CAD build for the part. Positions are in the model's coordinates, mm. Face numbers are marked on the shaded views. Give positions to 0.01 mm unless a question says otherwise; leave off trailing zeros. Order: outer loops, then holes, each group sorted by start corner. A loop starts at its lowest first (then second) coordinate and runs counter-clockwise, first axis right, second up.
Item 1: Wall check: L1, parallel to Z at x = -32.5, y = 0.8; L2, parallel to Z at x = 59.5, y = 0.85; L3, parallel to Z at x = 40, y = 1.95. Give the ranges that are in metal, low to high.
Item 2: Band-saw the part on A-A on z = -5.5. Give the cut face in (x, y), plus the area to 3 significant figures.
Item 3: Band-saw the part on D-D on x = 61. Give the cut face in (y, z).
Item 4: Band-saw the part on B-B on x = -25. Give the cut face in (y, z), plus the area to 3 significant figures.
Item 5: Flat gauge pin, fed straight in: P1, Ø0.6, axis at x = 65.5, y = 1, coming from the +Z side. Where does the tip first touch, or does it go through?
Item 6: Band-saw the part on C-C on y = 0.35. Give the cut face in (x, z).
Item 7: Two-plate mould, pull along Y, no slides. Class the marked faces 1 and 2: released by +Y, released by -Y, zero draft, split by the parting line, or undercut.
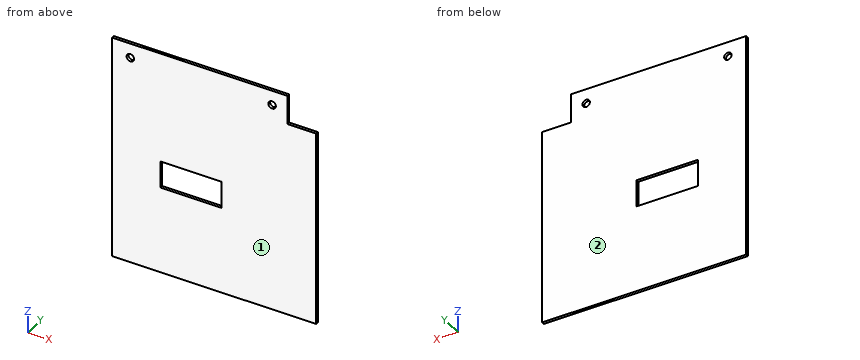
```python
from build123d import *

# Parameters (mm, degrees)
P_IDAT_VYSUNUT_M1_DEPTH  = 2
SKICA2_W                 = 42.685297449
SKICA2_H                 = 18.521827687
ODEBRAT_VYSUNUT_M1_DEPTH = 2
SKICA3_R                 = 2.6
ODEBRAT_VYSUNUT_M2_DEPTH = 2


with BuildPart() as part:
    # Skica1 → Přidat vysunutím1 (new body)
    with BuildSketch(Plane(origin=(0, 0, 0), x_dir=(1, 0, 0), z_dir=(0, 1, 0))):
        Polygon((51.954387959, -76.458238495), (-70.045612041, -76.458238495), (-70.045612041, 78.541761505), (71.954387959, 78.541761505), (71.954387959, -56.458238495), (51.954387959, -56.458238495), align=None)
    extrude(amount=P_IDAT_VYSUNUT_M1_DEPTH)

    # Skica2 → Odebrat vysunutím1 (cut)
    with BuildSketch(Plane(origin=(0, 2, 0), x_dir=(1, 0, 0), z_dir=(0, 1, 0))):
        with Locations((-15.127554213, 9.260913844)):
            Rectangle(SKICA2_W, SKICA2_H)
    extrude(amount=-ODEBRAT_VYSUNUT_M1_DEPTH, mode=Mode.SUBTRACT)

    # Skica3 → Odebrat vysunutím2 (cut)
    with BuildSketch(Plane.XZ):
        with Locations(Location((41.337845964, 66.458238495, 0), (0, 0, 270))):
            Circle(SKICA3_R)
        with Locations(Location((-57.3704334, 66.458238495, 0), (0, 0, 270))):
            Circle(SKICA3_R)
    extrude(amount=-ODEBRAT_VYSUNUT_M2_DEPTH, mode=Mode.SUBTRACT)


solid = part.part
```
The answers:
1. L1: z = -78.54 to -18.52, 0 to 76.46
1. L2: z = -78.54 to 56.46
1. L3: z = -78.54 to 64.23, 68.69 to 76.46
2. outline: (-70.05, 0) - (-36.47, 0) - (-36.47, 2) - (-70.05, 2) - close; (6.22, 0) - (71.95, 0) - (71.95, 2) - (6.22, 2) - close
2. area: 199 mm2
3. outline: (0, -78.54) - (2, -78.54) - (2, 56.46) - (0, 56.46) - close
4. outline: (0, -78.54) - (2, -78.54) - (2, -18.52) - (0, -18.52) - close; (0, 0) - (2, 0) - (2, 76.46) - (0, 76.46) - close
4. area: 273 mm2
5. P1: stops at z = 56.46
6. outline: (-70.05, -78.54) - (71.95, -78.54) - (71.95, 56.46) - (51.95, 56.46) - (51.95, 76.46) - (-70.05, 76.46) - close; hole circle Ø5.2 at (-57.37, 66.46); hole (-36.47, -18.52) - (6.22, -18.52) - (6.22, 0) - (-36.47, 0) - close; hole circle Ø5.2 at (41.34, 66.46)
7. face 1: released by -Y
7. face 2: released by +Y
